Read the model definition and answer for the solid it produces. Units are mm, in the model's axes. A direction names the side the tool comes from. Coordinates: 2 decimals unless noted, no trailing zeros. Loops run counter-clockwise (first coordinate to the right, second up) from the corner with the lowest first, then second, coordinate; pieces in that order, holes last. Notation, with made-up numbers: (44.25, 62) - (91.25, 62) arc R28 ccw to (91.25, 87) - close; hole circle Ø4 at (2.5, 69.25). An arc over 180 degrees is marked (long way). Use one line per item in the form item = value.
from build123d import *

# Parameters (mm, degrees)
IZIM1_W                     = 110
IZIM1_H                     = 50
Y_KSEKLIK_EKSTR_ZYON1_DEPTH = 3


with BuildPart() as part:
    # Çizim1 → Yükseklik-Ekstrüzyon1 (new body)
    with BuildSketch(Plane(origin=(0, 0, 0), x_dir=(1, 0, 0), z_dir=(0, 1, 0))):
        with Locations((55, -25)):
            Rectangle(IZIM1_W, IZIM1_H)
        with BuildLine():
            Line((20, -15), (90, -15))
            ThreePointArc((90, -15), (95, -20), (90, -25))
            Line((90, -25), (20, -25))
            ThreePointArc((20, -25), (15, -20), (20, -15))
        make_face(mode=Mode.SUBTRACT)
    extrude(amount=Y_KSEKLIK_EKSTR_ZYON1_DEPTH)


solid = part.part
Item 1: The part is cut by section C-C on z = 20. Give the vertices of the cut face in (x, y), plus the area to 3 significant figures.
Results below:
outline = (0, 0) - (15, 0) - (15, 3) - (0, 3) - close; (95, 0) - (110, 0) - (110, 3) - (95, 3) - close
area = 90.0 mm²
Item 2: Which of the six approach directions +Z, -Z, +X, -X, +Y, -Y give full straight-line access (tool end or side, diameter ignored) to faces 1 (the flat face through (55, 1, 15)), 2 (the flat face through (54, 0, 30))?
Results below:
face_1 = +Y, -Y
face_2 = +Z, -Z, +X, -X, -Y
Item 3: Find the intervals of material crossed by L1, parallel to Z at x = 57, y = 2.7; L2, parallel to Z at x = 93, y = 0.25, in increasing order.
Results below:
L1 = 0 to 15, 25 to 50
L2 = 0 to 16, 24 to 50
Item 4: The part is cut by section A-A on y = 1.7. Give the vertices of the cut face in (x, z).
Results below:
outline = (0, 0) - (110, 0) - (110, 50) - (0, 50) - close; hole (20, 15) - (90, 15) arc R5 ccw to (90, 25) - (20, 25) arc R5 ccw to start
Item 5: For a pull along X with two mould halves and no side action, classify faces 3 (the flat face through (110, 1, 25)), 4 (the flat face through (55, 1, 25)), 5 (the flat face through (54, 1, 0)) as +X half, -X half, draft (parallel to the pull), parting line (faces both ways), or undercut.
Results below:
face_3 = +X half
face_4 = undercut
face_5 = draft
Item 6: The part is cut by section B-B on x = 48. Give the vertices of the cut face in (y, z).
Results below:
outline = (0, 0) - (3, 0) - (3, 15) - (0, 15) - close; (0, 25) - (3, 25) - (3, 50) - (0, 50) - close
